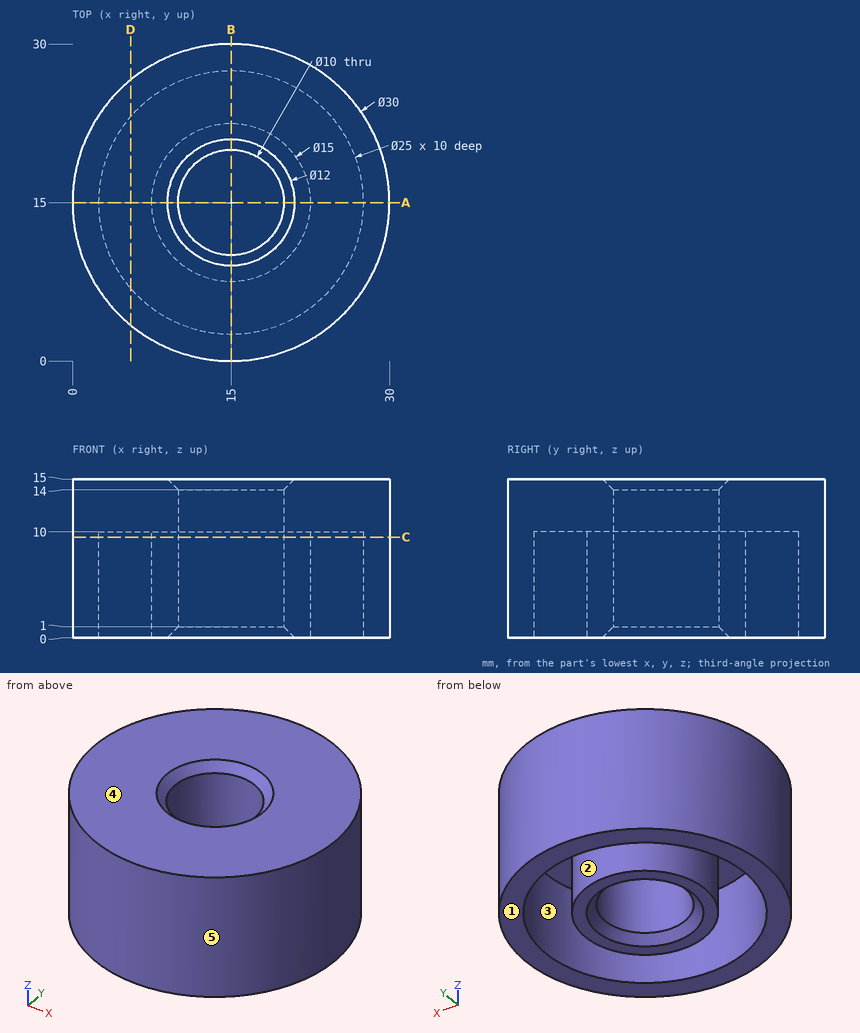
Answer from the drawing. Dimensions are ordinates in mm from the lowest x, y and z of the part. A direction names the side the tool comes from. Round coordinates to 2 decimals unless told otherwise and drop trailing zeros. Order: outer loops, then holes, each group sorted by start corner. A loop starts at its lowest first (then second) coordinate and runs counter-clockwise, first axis right, second up.
1) The part is cut by section D-D on x = 5.5. Write down the section's boundary in (y, z).
2) The part is cut by section C-C on z = 9.5. Write down the section's boundary in (x, y), plus the area to 3 significant figures.
3) Flat-ended cylindrical pins translate along their axes: pin 1 (3 mm diameter, centred on x = 15, y = 13, fed in from -Z); pin 2 (6 mm diameter, centred on y = 5, z = 7.5, fed in from +X); pin 3 (8 mm diameter, centred on x = 8, z = 5.5, fed in from +Y); pin 4 (1 mm diameter, centred on y = 25, z = 10.5, fed in from -X). Find the tip coordinate at first contact, or state that the pin passes through.
4) Straight lines are drawn through the part: L1, parallel to Y at x = 15, z = 9.25; L2, parallel to Y at x = 15, z = 10.75; L3, parallel to X at y = 16.5, z = 5. For each, find the intervals that lie inside material, in ascending order.
5) The part is cut by section A-A on y = 15. Write down the section's boundary in (x, z), plus the area to 3 significant figures.
6) For the marked faces 1 and 2, determine the directions among +Z, -Z, +X, -X, +Y, -Y from which every point of the face is accessible in a straight line to the end or side of a thin tool.
7) The mould has two halves that part along Y. Classify the marked faces 3, 4 and 5: released by +Y, released by -Y, zero draft, split by the parting line, or undercut.
Resolved:
1. outline: (3.39, 0) - (6.88, 0) - (6.88, 10) - (23.12, 10) - (23.12, 0) - (26.61, 0) - (26.61, 15) - (3.39, 15) - close
2. outline: circle Ø30 at (15, 15); circle Ø15 at (15, 15); hole circle Ø25 at (15, 15); hole circle Ø10 at (15, 15)
2. area: 314 mm2
3. pin 1: passes through
3. pin 2: stops at x = 28.27
3. pin 3: stops at y = 29.7
3. pin 4: stops at x = 3.39
4. L1: y = 0 to 2.5, 7.5 to 10, 20 to 22.5, 27.5 to 30
4. L2: y = 0 to 10, 20 to 30
4. L3: x = 0.08 to 2.59, 7.65 to 10.23, 19.77 to 22.35, 27.41 to 29.92
5. outline: (0, 0) - (2.5, 0) - (2.5, 10) - (7.5, 10) - (7.5, 0) - (9, 0) - (10, 1) - (10, 14) - (9, 15) - (0, 15) - close; (20, 1) - (21, 0) - (22.5, 0) - (22.5, 10) - (27.5, 10) - (27.5, 0) - (30, 0) - (30, 15) - (21, 15) - (20, 14) - close
5. area: 198 mm2
6. face 1: -Z, +X, -X, +Y, -Y
6. face 2: -Z
7. face 3: undercut
7. face 4: zero draft
7. face 5: split by the parting line
